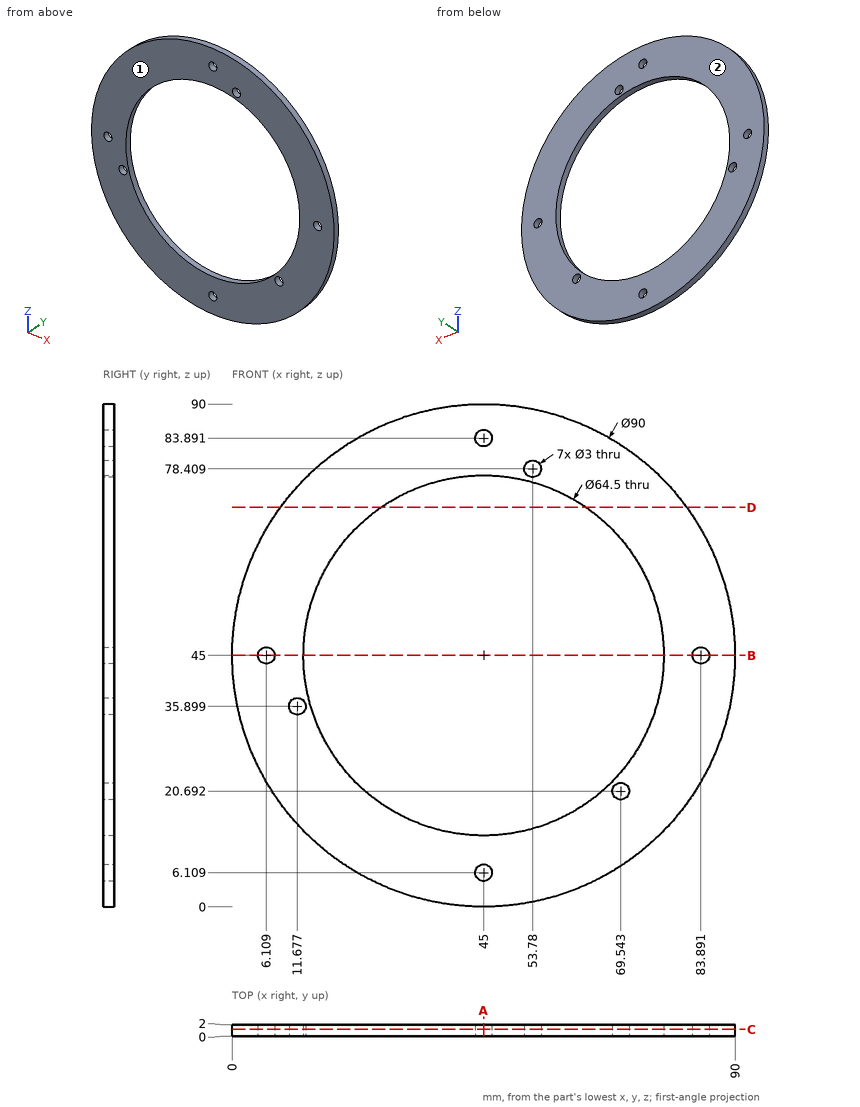
Source: three-view drawing plus pictorial views. Frame: mm from the lowest corner of the part. Coordinates: 2 decimals unless noted, no trailing zeros. Loops run counter-clockwise (first coordinate to the right, second up) from the corner with the lowest first, then second, coordinate; pieces in that order, holes last. Notation, with made-up numbers: (-33, 79.5) -> (16, 79.5) arc R12 cw to (16, 91.5) -> close; hole circle Ø1 at (36, 51.5). An arc over 180 degrees is marked (long way). Write each question's results on one line, items separated by ' | '. Start each with the question number.
Q1. Section D-D, the plane z = 71.5. Return the cut outline in (x, y).
Q2. Ray query, line 1 (X direction, y = 0.9, z = 45); line 2 (X direction, y = 1.3, z = 26.5) (1 decimal); line 3 (X direction, y = 1.9, z = 31) (1 decimal). Return the intervals inside material, ascending. Write a range as from..to.
Q3. Pull-direction query (Y, two-part tool) for the marked faces 1 and 2; classes: released by +Y, released by -Y, zero draft, split by the parting line, or undercut.
Q4. Section A-A, the plane x = 45. Return the cut outline in (y, z).
Q5. Section C-C, the plane y = 1.2. State how many separate pieces and enclosed holes the cut face has.
Q6. Section B-B, the plane z = 45. Return the cut outline in (x, y).
Q7. Pin query (flat end, axial travel): pin 1 (1.8 mm diameter, centred on x = 83.89, z = 45, fed in from -Y); pin 2 (1 mm diameter, centred on x = 26, y = 1.5, fed in from -Z); pin 3 (1 mm diameter, centred on x = 63, y = 1.5, fed in from -Z). Return the tip coordinate at first contact, or that it passes through.
Found:
1) outline: (8.63, 0) -> (26.62, 0) -> (26.62, 2) -> (8.63, 2) -> close; (63.38, 0) -> (81.37, 0) -> (81.37, 2) -> (63.38, 2) -> close
2) line 1: 0..4.61, 7.61..12.75, 77.25..82.39, 85.39..90 | line 2: 4..18.6, 71.4..86 | line 3: 2.2..15.9, 74.1..87.8
3) face 1: released by -Y | face 2: released by +Y
4) outline: (0, 0) -> (2, 0) -> (2, 4.61) -> (0, 4.61) -> close; (0, 7.61) -> (2, 7.61) -> (2, 12.75) -> (0, 12.75) -> close; (0, 77.25) -> (2, 77.25) -> (2, 82.39) -> (0, 82.39) -> close; (0, 85.39) -> (2, 85.39) -> (2, 90) -> (0, 90) -> close
5) separate pieces: 1 | enclosed holes: 8
6) outline: (0, 0) -> (4.61, 0) -> (4.61, 2) -> (0, 2) -> close; (7.61, 0) -> (12.75, 0) -> (12.75, 2) -> (7.61, 2) -> close; (77.25, 0) -> (82.39, 0) -> (82.39, 2) -> (77.25, 2) -> close; (85.39, 0) -> (90, 0) -> (90, 2) -> (85.39, 2) -> close
7) pin 1: through | pin 2: z = 3.98 | pin 3: z = 3.54
